Geometry: final body of the model. Coordinates: model frame, mm. Face numbers are marked on the shaded views. A direction names the side the tool comes from. Give positions to 0.01 mm unless a question says otherwise; leave off trailing zeros. Write each loop counter-clockwise with the first axis right and the second up, starting at its lowest first coordinate (ties: lowest second). Pieces come first, ordered by that corner, then holes. Notation, with made-up numbers: M 46,38 L 88,38 A8 ccw 88,53 Z; hole C -30.75,-36.75 d3. An arc over 180 degrees is marked long. Use a Markdown table: item, result. Add a question column.
1) Pin query (flat end, axial travel): pin 1 (3 mm diameter, centred on x = -41, z = 3.5, fed in from +Y); pin 2 (1 mm diameter, centred on x = -18.5, z = 2.5, fed in from -Y); pin 3 (1 mm diameter, centred on y = 21.5, z = 0.5, fed in from -X). Return the tip coordinate at first contact, or that it passes through.
2) Section D-D on x = -13.5. Return the cut outline in (y, z).
3) Section C-C on z = 3.45. State how many separate pieces and enclosed holes the cut face has, then the cut area to 3 significant figures.
4) Section A-A on y = 15.5. Return the cut outline in (x, z), then the cut area to 3 significant figures.
5) Draft query along X for the marked faces 1, 2 and 3. Return one class per face: +X half, -X half, draft (parallel to the pull), parting line (faces both ways), or undercut.
6) Section B-B on x = -31. Return the cut outline in (y, z).
7) Set-up query: the marked faces 4, 5 and 6. Return all of +Z, -Z, +X, -X, +Y, -Y with unobstructed straight access to the full face (end or side cutting, diameter ignored); none if empty.
8) Line query: line 1 (X direction, y = 15.75, z = 5.2); line 2 (Y direction, x = -5.5, z = 2.15); line 3 (Y direction, x = -20, z = 3.65). Output: solid intervals per line, ascending.
```python
from build123d import *

# Parameters (mm, degrees)
BOSS_EXTRUDE1_DEPTH = 5.842


with BuildPart() as part:
    # Sketch1 → Boss-Extrude1 (new body)
    with BuildSketch(Plane.XY):
        with BuildLine():
            Line((0, 0), (-6.35, 0))
            ThreePointArc((-6.35, 0), (-8.948239117, 0.689575054), (-10.086248608, 3.125))
            ThreePointArc((-10.086248608, 3.125), (-10.825823663, 5.161990509), (-12.7, 6.25))
            Line((-12.7, 6.25), (-25.4, 6.25))
            ThreePointArc((-25.4, 6.25), (-27.274176337, 5.161990509), (-28.013751392, 3.125))
            ThreePointArc((-28.013751392, 3.125), (-29.151760883, 0.689575054), (-31.75, 0))
            Line((-31.75, 0), (-38.1, 0))
            Line((-38.1, 0), (-38.1, 6.25))
            Line((-38.1, 6.25), (-43.942, 6.25))
            Line((-43.942, 6.25), (-43.942, 19.15))
            Line((-43.942, 19.15), (-38.1, 19.15))
            Line((-38.1, 19.15), (-38.1, 25.4))
            Line((-38.1, 25.4), (0, 25.4))
            Line((0, 25.4), (0, 19.15))
            Line((0, 19.15), (5.842, 19.15))
            Line((5.842, 19.15), (5.842, 6.25))
            Line((5.842, 6.25), (0, 6.25))
            Line((0, 6.25), (0, 0))
        make_face()
        with BuildLine():
            Line((-4.621403, 12.844653), (-8.078597, 12.844653))
            ThreePointArc((-8.078597, 12.844653), (-8.437807245, 12.993442755), (-8.586597, 13.352653))
            Line((-8.586597, 13.352653), (-8.586597, 16.809847))
            ThreePointArc((-8.586597, 16.809847), (-8.437807245, 17.169057245), (-8.078597, 17.317847))
            Line((-8.078597, 17.317847), (-4.621403, 17.317847))
            ThreePointArc((-4.621403, 17.317847), (-4.262192755, 17.169057245), (-4.113403, 16.809847))
            Line((-4.113403, 16.809847), (-4.113403, 13.352653))
            ThreePointArc((-4.113403, 13.352653), (-4.262192755, 12.993442755), (-4.621403, 12.844653))
        make_face(mode=Mode.SUBTRACT)
        with BuildLine():
            Line((-16.813403, 13.352653), (-16.813403, 16.809847))
            ThreePointArc((-16.813403, 16.809847), (-16.962192755, 17.169057245), (-17.321403, 17.317847))
            Line((-17.321403, 17.317847), (-20.778597, 17.317847))
            ThreePointArc((-20.778597, 17.317847), (-21.137807245, 17.169057245), (-21.286597, 16.809847))
            Line((-21.286597, 16.809847), (-21.286597, 13.352653))
            ThreePointArc((-21.286597, 13.352653), (-21.137807245, 12.993442755), (-20.778597, 12.844653))
            Line((-20.778597, 12.844653), (-17.321403, 12.844653))
            ThreePointArc((-17.321403, 12.844653), (-16.962192755, 12.993442755), (-16.813403, 13.352653))
        make_face(mode=Mode.SUBTRACT)
        with BuildLine():
            Line((-29.513403, 13.352653), (-29.513403, 16.809847))
            ThreePointArc((-29.513403, 16.809847), (-29.662192755, 17.169057245), (-30.021403, 17.317847))
            Line((-30.021403, 17.317847), (-33.478597, 17.317847))
            ThreePointArc((-33.478597, 17.317847), (-33.837807245, 17.169057245), (-33.986597, 16.809847))
            Line((-33.986597, 16.809847), (-33.986597, 13.352653))
            ThreePointArc((-33.986597, 13.352653), (-33.837807245, 12.993442755), (-33.478597, 12.844653))
            Line((-33.478597, 12.844653), (-30.021403, 12.844653))
            ThreePointArc((-30.021403, 12.844653), (-29.662192755, 12.993442755), (-29.513403, 13.352653))
        make_face(mode=Mode.SUBTRACT)
    extrude(amount=BOSS_EXTRUDE1_DEPTH)


solid = part.part
```
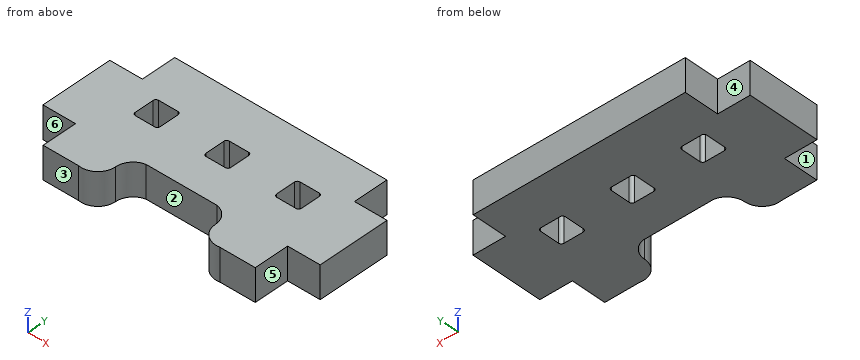
Found:
| question | item | result |
|---|---|---|
| 1 | pin 1 | y = 19.15 |
| 1 | pin 2 | y = 6.25 |
| 1 | pin 3 | x = -38.1 |
| 2 | outline | M 6.25,0 L 25.4,0 L 25.4,5.84 L 6.25,5.84 Z |
| 3 | separate pieces | 1 |
| 3 | enclosed holes | 3 |
| 3 | area | 947 mm² |
| 4 | outline | M -43.94,0 L -33.99,0 L -33.99,5.84 L -43.94,5.84 Z; M -29.51,0 L -21.29,0 L -21.29,5.84 L -29.51,5.84 Z; M -16.81,0 L -8.59,0 L -8.59,5.84 L -16.81,5.84 Z; M -4.11,0 L 5.84,0 L 5.84,5.84 L -4.11,5.84 Z |
| 4 | area | 212 mm² |
| 5 | face 1 | -X half |
| 5 | face 2 | undercut |
| 5 | face 3 | draft |
| 6 | outline | M -0.04,0 L 12.84,0 L 12.84,5.84 L -0.04,5.84 Z; M 17.32,0 L 25.4,0 L 25.4,5.84 L 17.32,5.84 Z |
| 7 | face 4 | +Z, -Z, -X, +Y |
| 7 | face 5 | +Z, -Z, +X, -Y |
| 7 | face 6 | +Z, -Z, -X, -Y |
| 8 | line 1 | -43.94 to -33.99, -29.51 to -21.29, -16.81 to -8.59, -4.11 to 5.84 |
| 8 | line 2 | 0 to 12.84, 17.32 to 25.4 |
| 8 | line 3 | 6.25 to 12.84, 17.32 to 25.4 |
